```python
from build123d import *

# Parameters (mm, degrees)
SKETCH2_R           = 27
SKETCH2_R_2         = 2.125
BOSS_EXTRUDE2_DEPTH = 10
SKETCH3_R           = 3.275
CUT_EXTRUDE1_DEPTH  = 7.5
CUT_EXTRUDE2_START  = -5
SKETCH4_R           = 27
SKETCH4_R_2         = 5.275
CUT_EXTRUDE2_DEPTH  = 5
SKETCH5_W           = 8.128
SKETCH5_H           = 8.13
CUT_EXTRUDE3_DEPTH  = 3.2


with BuildPart() as part:
    # Sketch2 → Boss-Extrude2 (new body)
    with BuildSketch(Plane(origin=(0, 0, 0), x_dir=(1, 0, 0), z_dir=(0, 1, 0))):
        with Locations(Location((0, 0, 0), (0, 0, 270))):
            Circle(SKETCH2_R)
        with Locations(Location((0, 0, 0), (0, 0, 270))):
            Circle(SKETCH2_R_2, mode=Mode.SUBTRACT)
    extrude(amount=BOSS_EXTRUDE2_DEPTH)

    # Sketch3 → Cut-Extrude1 (cut)
    with BuildSketch(Plane.XZ.offset(-10)):
        with Locations(Location((9.52625, -16.499949006, 0), (0, 0, 270))):
            Circle(SKETCH3_R)
        with Locations(Location((9.52625, 16.499949006, 0), (0, 0, 270))):
            Circle(SKETCH3_R)
        with Locations(Location((-19.0525, 0, 0), (0, 0, 270))):
            Circle(SKETCH3_R)
    extrude(amount=CUT_EXTRUDE1_DEPTH, mode=Mode.SUBTRACT)

    # Sketch4 → Cut-Extrude2 (cut)
    with BuildSketch(Plane(origin=(0, 10, 0), x_dir=(1, 0, 0), z_dir=(0, 1, 0)).offset(CUT_EXTRUDE2_START)):
        with Locations(Location((0, 0, 0), (0, 0, 270))):
            Circle(SKETCH4_R)
        with Locations(Location((-19.0525, 0, 0), (0, 0, 270))):
            Circle(SKETCH4_R_2, mode=Mode.SUBTRACT)
        with Locations(Location((9.52625, -16.499949006, 0), (0, 0, 270))):
            Circle(SKETCH4_R_2, mode=Mode.SUBTRACT)
        with Locations(Location((9.52625, 16.499949006, 0), (0, 0, 270))):
            Circle(SKETCH4_R_2, mode=Mode.SUBTRACT)
    extrude(amount=CUT_EXTRUDE2_DEPTH, mode=Mode.SUBTRACT)

    # Sketch5 → Cut-Extrude3 (cut)
    with BuildSketch(Plane.XZ):
        Rectangle(SKETCH5_W, SKETCH5_H)
    extrude(amount=-CUT_EXTRUDE3_DEPTH, mode=Mode.SUBTRACT)


solid = part.part
```
Check sheet for the modelled part. Datum: model origin and axes. Units: mm. A direction names the side the tool comes from. Round coordinates to 2 decimals unless told otherwise and drop trailing zeros. Loops run counter-clockwise (first coordinate to the right, second up) from the corner with the lowest first, then second, coordinate; pieces in that order, holes last. Notation, with made-up numbers: M 30,75 L 78,75 A13 ccw 78,85 Z; hole C -16,70.25 d7. An arc over 180 degrees is marked long. Answer as a JSON object with one key per item and string values.
1. Section check C-C (y = 6.75). State how many separate pieces and enclosed holes the cut face has, plus the area to 3 significant figures.
Reply:
{"separate pieces": "3", "enclosed holes": "3", "area": "161 mm²"}
2. Gauge pin test, flat ends, axial feed: P1, Ø1.5, axis at y = 6.5, z = 4, coming from the +X side; P2, Ø1.6, axis at x = 1.5, y = 1.5, coming from the +Z side; P3, Ø1, axis at y = 5, z = 2, coming from the +X side. Record the tip position at first contact, or that the pin passes through.
Reply:
{"P1": "stops at x = -14.9", "P2": "stops at z = 26.99", "P3": "stops at x = 26.96"}
3. Mould release check, pull along X, two halves, no side actions. Record for faces 4 (the cylindrical face through (12.773, 6.302, -16.074)), 5 (the flat face through (0, 5, 6)), 6 (the cylindrical face through (9.67, 6.3, 19.77)), 7 (the cylindrical face through (-13.822, 7.465, -0.687)): pulls with the +X half, pulls with the -X half, needs draft (parallel to the pull), parting line crosses it, or undercut.
Reply:
{"face 4": "undercut", "face 5": "needs draft", "face 6": "undercut", "face 7": "parting line crosses it"}
4. Section check B-B (x = 0). Record the boundary of the cut face in (y, z) (3 decimals).
Reply:
{"outline": "M 0,-27 L 5,-27 L 5,-2.125 L 3.2,-2.125 L 3.2,-4.065 L 0,-4.065 Z; M 0,4.065 L 3.2,4.065 L 3.2,2.125 L 5,2.125 L 5,27 L 0,27 Z"}
5. Scan lines: line 1 (X direction, y = 4.1, z = 0) (1 decimal); line 2 (X direction, y = 2.75, z = 1.5); line 3 (Y direction, x = 13.5, z = 12.5). Record each from-to range of solid material in increasing order.
Reply:
{"line 1": "x = -27 to -22.3, -15.8 to -2.1, 2.1 to 27", "line 2": "x = -26.96 to -21.96, -16.14 to -4.06, 4.06 to 26.96", "line 3": "y = 0 to 5"}
6. Section check D-D (y = 1.5). Record the boundary of the cut face in (x, z) (3 decimals), plus the area to 3 significant figures.
Reply:
{"outline": "C 0,0 d54; hole M -4.064,-4.065 L 4.064,-4.065 L 4.064,4.065 L -4.064,4.065 Z", "area": "2,220 mm²"}
7. Section check A-A (z = 0). Record the boundary of the cut face in (x, y) (1 decimal), plus the area to 3 significant figures.
Reply:
{"outline": "M -27,0 L -4.1,0 L -4.1,3.2 L -2.1,3.2 L -2.1,5 L -13.8,5 L -13.8,10 L -15.8,10 L -15.8,2.5 L -22.3,2.5 L -22.3,10 L -24.3,10 L -24.3,5 L -27,5 Z; M 2.1,3.2 L 4.1,3.2 L 4.1,0 L 27,0 L 27,5 L 2.1,5 Z", "area": "240 mm²"}
8. Access from +Z, -Z, +X, -X, +Y, -Y to the whole of each face (thin tool, end or side, straight path). Record for faces 1 (the flat face through (-4.064, 2, 0)), 2 (the flat face through (12, 10, 19)), 3 (the cylindrical face through (-22.25, 6.3, 0.71)).
Reply:
{"face 1": "-Y", "face 2": "+Z, -Z, +X, -X, +Y", "face 3": "+Y"}
